Build history of the part. All positions in model axes, mm. A direction names the side the tool comes from. Coordinates: 2 decimals unless noted, no trailing zeros. Order: outer loops, then holes, each group sorted by start corner. A loop starts at its lowest first (then second) coordinate and runs counter-clockwise, first axis right, second up. Notation, with made-up numbers: (13.5, 40.25) - (18.5, 40.25) arc R10 ccw to (18.5, 57.25) - close; hole circle Ø8 at (70, 57.25). An arc over 180 degrees is marked (long way). One line per item, written item: value.
from build123d import *

# Parameters (mm, degrees)
SKETCH1_W                = 15.24
SKETCH1_H                = 6.35
BOSS_EXTRUDE1_DEPTH      = 21.59
SKETCH2_W                = 15.24
SKETCH2_H                = 5.08
BOSS_EXTRUDE2_DEPTH      = 29.21
M3_CLEARANCE_HOLE1_D     = 3.7
M3_CLEARANCE_HOLE1_DEPTH = 25.4
M3_CLEARANCE_HOLE1_TIP   = 1.111592145
M3_CLEARANCE_HOLE2_D     = 3.7
M3_CLEARANCE_HOLE2_DEPTH = 25.4
M3_CLEARANCE_HOLE2_TIP   = 1.111592145


with BuildPart() as part:
    # Sketch1 → Boss-Extrude1 (new body)
    with BuildSketch(Plane(origin=(0, 0, 0), x_dir=(1, 0, 0), z_dir=(0, 1, 0))):
        with Locations((0, -1.264380531)):
            Rectangle(SKETCH1_W, SKETCH1_H)
    extrude(amount=BOSS_EXTRUDE1_DEPTH)

    # Sketch2 → Boss-Extrude2 (add)
    with BuildSketch(Plane.XY.offset(4.439380531)):
        with Locations((0, 2.54)):
            Rectangle(SKETCH2_W, SKETCH2_H)
    extrude(amount=BOSS_EXTRUDE2_DEPTH)

    # M3 Clearance Hole1
    with Locations(Plane(origin=(0, 5.08, 0), x_dir=(1, 0, 0), z_dir=(0, 1, 0))):
        with Locations((0, -28.061380531)):
            Hole(M3_CLEARANCE_HOLE1_D / 2, depth=M3_CLEARANCE_HOLE1_DEPTH)
            with Locations((0, 0, -(M3_CLEARANCE_HOLE1_DEPTH + M3_CLEARANCE_HOLE1_TIP / 2))):  # 118° drill point
                Cone(0, M3_CLEARANCE_HOLE1_D / 2, M3_CLEARANCE_HOLE1_TIP, mode=Mode.SUBTRACT)

    # M3 Clearance Hole2
    with Locations(Plane.XY.offset(4.439380531)):
        with Locations((0, 18.288)):
            Hole(M3_CLEARANCE_HOLE2_D / 2, depth=M3_CLEARANCE_HOLE2_DEPTH)
            with Locations((0, 0, -(M3_CLEARANCE_HOLE2_DEPTH + M3_CLEARANCE_HOLE2_TIP / 2))):  # 118° drill point
                Cone(0, M3_CLEARANCE_HOLE2_D / 2, M3_CLEARANCE_HOLE2_TIP, mode=Mode.SUBTRACT)


solid = part.part
1. Band-saw the part on C-C, the plane y = 9. Give the cut face in (x, z).
Values found:
outline: (-7.62, -1.91) - (7.62, -1.91) - (7.62, 4.44) - (-7.62, 4.44) - close
2. Band-saw the part on D-D, the plane z = 15.5. Give the cut face in (x, y).
Values found:
outline: (-7.62, 0) - (7.62, 0) - (7.62, 5.08) - (-7.62, 5.08) - close
3. Two-plate mould, pull along X, no slides. Class faces 3 (the face through (7.62, 3, 8)), 4 (the face through (0.241, 2.504, 26.227)), 5 (the face through (0, 3, 33.649)): pulls with the +X half, pulls with the -X half, needs draft (parallel to the pull), parting line crosses it, or undercut.
Values found:
face 3: pulls with the +X half
face 4: undercut
face 5: needs draft
4. Probe line 1 along Z through (x, y) = (0, 3.8); line 2 along Y through (x, z) = (0, 1); line 3 along Z through (x, y) = (-6.25, 6). List the from-to ranges inside material, lowest first.
Values found:
line 1: z = -1.91 to 26.21, 29.91 to 33.65
line 2: y = 0 to 16.44, 20.14 to 21.59
line 3: z = -1.91 to 4.44
5. Band-saw the part on A-A, the plane x = 0. Give the cut face in (y, z), and give its area (3 significant figures).
Values found:
outline: (0, -1.91) - (16.44, -1.91) - (16.44, 4.44) - (5.08, 4.44) - (5.08, 26.21) - (0, 26.21) - close; (0, 29.91) - (5.08, 29.91) - (5.08, 33.65) - (0, 33.65) - close; (20.14, -1.91) - (21.59, -1.91) - (21.59, 4.44) - (20.14, 4.44) - close
area: 243 mm2
6. 3-axis set-ups, long thin cutter, end or side, ignore diameter. For faces 1 (the face through (0, 21.59, 1)), 2 (the face through (0, 5.08, 19)): which of +Z, -Z, +X, -X, +Y, -Y reach the whole face in a straight line?
Values found:
face 1: +Z, -Z, +X, -X, +Y
face 2: +Z, +X, -X, +Y
7. Band-saw the part on B-B, the plane x = 6. Give the cut face in (y, z), and give its area (3 significant figures).
Values found:
outline: (0, -1.91) - (21.59, -1.91) - (21.59, 4.44) - (5.08, 4.44) - (5.08, 33.65) - (0, 33.65) - close
area: 285 mm2
8. Flat gauge pins, fed straight in: P1, Ø6, axis at x = -1, z = 16, coming from the +Y side; P2, Ø4, axis at x = -2, z = 8, coming from the -Y side. Where does each tip first touch, or does it go through?
Values found:
P1: stops at y = 5.08
P2: stops at y = 0
